```python
from build123d import *

# Parameters (mm, degrees)
SM_BASE_FLANGE_1_DEPTH = 131.5
HOLE_WIZARD_M6_1_D     = 7
SKETCH_6_W             = 80.4
SKETCH_6_H             = 40
CUT_EXTRUDE_1_DEPTH    = 248.738773711
HOLE_WIZARD_M5_1_D     = 4.2
OTHER_START            = 172.5
OTHER_1_DEPTH          = 1.5


# Read off the part's stored shape, not the designer's step: 断开-边角1
# Sheet-metal steps are written as plain solids
with BuildPart() as part:
    # Sketch 1 → 基体-法兰1 (new, symmetric)
    with BuildSketch(Plane(origin=(0, 0, 0), x_dir=(0, 0, -1), z_dir=(1, 0, 0))):
        with BuildLine():
            Line((0, 0), (0, 171.5))
            ThreePointArc((0, 171.5), (0.732233047, 173.267766953), (2.5, 174))
            Line((2.5, 174), (117.5, 174))
            Line((117.5, 174), (117.5, 172.5))
            Line((117.5, 172.5), (2.5, 172.5))
            ThreePointArc((2.5, 172.5), (1.792893219, 172.207106781), (1.5, 171.5))
            Line((1.5, 171.5), (1.5, 0))
            Line((1.5, 0), (0, 0))
        make_face()
    extrude(amount=SM_BASE_FLANGE_1_DEPTH, both=True)

    # M6 间隙孔1 (through all)
    with Locations(Plane(origin=(0, 0, -1.5), x_dir=(-1, 0, 0), z_dir=(0, 0, -1))):
        with Locations((-99, 75), (-99, 35), (99, 35), (99, 75)):
            Hole(HOLE_WIZARD_M6_1_D / 2)

    # 草图6 → 切除-拉伸1 (cut, through all)
    with BuildSketch(Plane.XY):
        with Locations((0, 20)):
            Rectangle(SKETCH_6_W, SKETCH_6_H)
    extrude(amount=-CUT_EXTRUDE_1_DEPTH, mode=Mode.SUBTRACT)

    # M5 螺纹孔1 (through all)
    with Locations(Plane(origin=(0, 174, 0), x_dir=(1, 0, 0), z_dir=(0, 1, 0))):
        with Locations((9, 107), (31.5, 107), (31.5, 42), (9, 42)):
            Hole(HOLE_WIZARD_M5_1_D / 2)

    # Other 1 outline → Other 1 (cut)
    with BuildSketch(Plane(origin=(0, 0, 0), x_dir=(1, 0, 0), z_dir=(0, 1, 0)).offset(OTHER_START)):
        with BuildLine():
            Line((131.5, 117.5), (129.5, 117.5))
            ThreePointArc((129.5, 117.5), (130.914213562, 116.914213562), (131.5, 115.5))
            Line((131.5, 115.5), (131.5, 117.5))
        make_face()
        with BuildLine():
            ThreePointArc((-131.5, 115.5), (-130.914213562, 116.914213562), (-129.5, 117.5))
            Line((-129.5, 117.5), (-131.5, 117.5))
            Line((-131.5, 117.5), (-131.5, 115.5))
        make_face()
    extrude(amount=OTHER_1_DEPTH, mode=Mode.SUBTRACT)


solid = part.part
```
Check sheet for the modelled part. Datum: model origin and axes. Units: mm. A direction names the side the tool comes from. Give positions to 0.01 mm unless a question says otherwise; leave off trailing zeros. Order: outer loops, then holes, each group sorted by start corner. A loop starts at its lowest first (then second) coordinate and runs counter-clockwise, first axis right, second up. Notation, with made-up numbers: (47.5, -22) -> (57.5, -22) arc R11 ccw to (57.5, -9) -> close; hole circle Ø7 at (56, 0.5). An arc over 180 degrees is marked (long way). Return JSON: item names as keys, results as strings.
1. Cross-section at D-D, the plane z = -97.5. Record the cut outline in (x, y).
From the geometry:
{"outline": "(-131.5, 172.5) -> (131.5, 172.5) -> (131.5, 174) -> (-131.5, 174) -> close"}
2. Cross-section at C-C, the plane x = 105.5. Record the cut outline in (y, z), plus the area to 3 significant figures.
From the geometry:
{"outline": "(0, -1.5) -> (171.5, -1.5) arc R1 cw to (172.5, -2.5) -> (172.5, -117.5) -> (174, -117.5) -> (174, -2.5) arc R2.5 ccw to (171.5, 0) -> (0, 0) -> close", "area": "434 mm^2"}
3. Cross-section at B-B, the plane x = -99. Record the cut outline in (y, z), plus the area to 3 significant figures.
From the geometry:
{"outline": "(0, -1.5) -> (31.5, -1.5) -> (31.5, 0) -> (0, 0) -> close; (38.5, -1.5) -> (71.5, -1.5) -> (71.5, 0) -> (38.5, 0) -> close; (78.5, -1.5) -> (171.5, -1.5) arc R1 cw to (172.5, -2.5) -> (172.5, -117.5) -> (174, -117.5) -> (174, -2.5) arc R2.5 ccw to (171.5, 0) -> (78.5, 0) -> close", "area": "413 mm^2"}
4. Material ranges on probe 1 along X at (y, z) = (173.3, -42); probe 2 along Y at (x, z) = (-99, -0.8); probe 3 along Z at (x, y) = (9, 173.4), recorded low to high. Write a range as [from, to].
From the geometry:
{"probe 1": "[-131.5, 6.9], [11.1, 29.4], [33.6, 131.5]", "probe 2": "[0, 31.5], [38.5, 71.5], [78.5, 173.33]", "probe 3": "[-117.5, -109.1], [-104.9, -44.1], [-39.9, -0.88]"}
5. Set-up check for faces 3 (the flat face through (2, 87, -1.5)), 4 (the cylindrical face through (-95.767, 73.659, -0.74)): record each of +Z, -Z, +X, -X, +Y, -Y from which the full face is reachable in a straight line by a thin tool's end or side.
From the geometry:
{"face 3": "-Z, +X, -X, -Y", "face 4": "+Z, -Z"}
6. Cross-section at A-A, the plane y = 20. Record the cut outline in (x, z).
From the geometry:
{"outline": "(-131.5, -1.5) -> (-40.2, -1.5) -> (-40.2, 0) -> (-131.5, 0) -> close; (40.2, -1.5) -> (131.5, -1.5) -> (131.5, 0) -> (40.2, 0) -> close"}
7. Mould release check, pull along X, two halves, no side actions. Record for faces 1 (the flat face through (2, 172.5, -61)), 2 (the cylindrical face through (102.34, 36.05, -0.74)): +X half, -X half, draft (parallel to the pull), parting line (faces both ways), or undercut.
From the geometry:
{"face 1": "draft", "face 2": "undercut"}
8. Go/stop test with flat-tipped pins: P1, Ø4, axis at x = 62.5, z = -99.5, coming from the -Y side; P2, Ø12, axis at x = -56.5, y = 147, coming from the -Z side; P3, Ø1.6, axis at x = 2, z = -1, coming from the -Y side; P4, Ø11, axis at x = 99, y = 75, coming from the +Z side. Record where each tip stops, or that it passes through.
From the geometry:
{"P1": "y = 172.5", "P2": "z = -1.5", "P3": "y = 40", "P4": "z = 0"}
